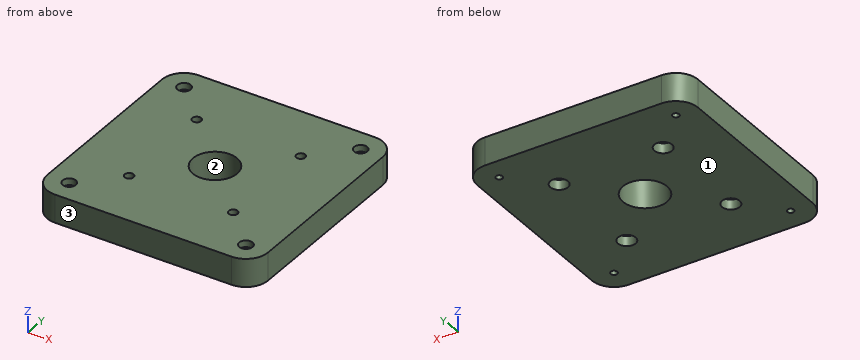
from build123d import *

# Parameters (mm, degrees)
SALIENTE_EXTRUIR4_START = 70
SALIENTE_EXTRUIR4_DEPTH = 12.7
CROQUIS8_R              = 3
CORTAR_EXTRUIR1_DEPTH   = 3
CROQUIS13_R             = 1.5
CORTAR_EXTRUIR4_DEPTH   = 30
CROQUIS16_R             = 10
CROQUIS16_R_2           = 2
CORTAR_EXTRUIR6_DEPTH   = 31
CROQUIS21_R             = 4
CORTAR_EXTRUIR12_DEPTH  = 4.5


with BuildPart() as part:
    # Croquis5 → Saliente-Extruir4 (new body)
    with BuildSketch(Plane.XY.offset(12.7).offset(SALIENTE_EXTRUIR4_START)):
        with BuildLine():
            Line((160, 0), (80, 0))
            ThreePointArc((80, 0), (72.928932188, 2.928932188), (70, 10))
            Line((70, 10), (70, 90))
            ThreePointArc((70, 90), (72.928932188, 97.071067812), (80, 100))
            Line((80, 100), (160, 100))
            ThreePointArc((160, 100), (167.071067812, 97.071067812), (170, 90))
            Line((170, 90), (170, 10))
            ThreePointArc((170, 10), (167.071067812, 2.928932188), (160, 0))
        make_face()
    extrude(amount=SALIENTE_EXTRUIR4_DEPTH)

    # Croquis8 → Cortar-Extruir1 (cut)
    with BuildSketch(Plane.XY.offset(95.4)):
        with Locations((80, 90)):
            Circle(CROQUIS8_R)
        with Locations((160, 90)):
            Circle(CROQUIS8_R)
        with Locations((160, 10)):
            Circle(CROQUIS8_R)
        with Locations((80, 10)):
            Circle(CROQUIS8_R)
    extrude(amount=-CORTAR_EXTRUIR1_DEPTH, mode=Mode.SUBTRACT)

    # Croquis13 → Cortar-Extruir4 (cut)
    with BuildSketch(Plane.XY.offset(95.4)):
        with Locations((80, 90)):
            Circle(CROQUIS13_R)
        with Locations((160, 90)):
            Circle(CROQUIS13_R)
        with Locations((160, 10)):
            Circle(CROQUIS13_R)
        with Locations((80, 10)):
            Circle(CROQUIS13_R)
    extrude(amount=-CORTAR_EXTRUIR4_DEPTH, mode=Mode.SUBTRACT)

    # Croquis16 → Cortar-Extruir6 (cut)
    with BuildSketch(Plane.XY.offset(95.4)):
        with Locations((120, 50)):
            Circle(CROQUIS16_R)
        with Locations((96.43, 73.57)):
            Circle(CROQUIS16_R_2)
        with Locations((143.57, 73.57)):
            Circle(CROQUIS16_R_2)
        with Locations((96.43, 26.43)):
            Circle(CROQUIS16_R_2)
        with Locations((143.57, 26.43)):
            Circle(CROQUIS16_R_2)
    extrude(amount=-CORTAR_EXTRUIR6_DEPTH, mode=Mode.SUBTRACT)

    # Croquis21 → Cortar-Extruir12 (cut)
    with BuildSketch(Plane(origin=(0, 0, 82.7), x_dir=(-1, 0, 0), z_dir=(0, 0, -1))):
        with Locations((-143.57, 73.57)):
            Circle(CROQUIS21_R)
        with Locations((-96.43, 73.57)):
            Circle(CROQUIS21_R)
        with Locations((-143.57, 26.43)):
            Circle(CROQUIS21_R)
        with Locations((-96.43, 26.43)):
            Circle(CROQUIS21_R)
    extrude(amount=-CORTAR_EXTRUIR12_DEPTH, mode=Mode.SUBTRACT)


solid = part.part
For this review, take the finished solid that the model builds, in its own axes (mm). Face numbers are marked on the shaded views. Round coordinates to 2 decimals unless told otherwise and drop trailing zeros. Write each loop counter-clockwise with the first axis right and the second up, starting at its lowest first coordinate (ties: lowest second). Pieces come first, ordered by that corner, then holes. Notation, with made-up numbers: (4.5, 7) - (62.5, 7) arc R30 ccw to (62.5, 43) - close; hole circle Ø3 at (41, -21). An arc over 180 degrees is marked (long way). Write item = value, one per line. Start each with the question number.
1. Consider section D-D on z = 85.25. Give the number of separate pieces and of enclosed holes in the cut face, plus the area to 3 significant figures.
2. Consider section B-B on y = 50. State the section outline as (x, z) points, plus the area to 3 significant figures.
3. Consider section A-A on x = 96.43. State the section outline as (y, z) points.
4. Consider section C-C on y = 73.57. State the section outline as (x, z) points.
5. For pin 1 Ø10.5 at (x, y) = (96.43, 73.57) entering from -Z; pin 2 Ø4 at (x, y) = (97, 73.5) entering from -Z; pin 3 Ø12 at (x, y) = (120, 50) entering from +Z; pin 4 Ø1.8 at (x, y) = (81, 10.5) entering from +Z, all flat-tipped, find the tip position at first contact; note any pin that passes through.
6. Wall thickness on L1, parallel to Y at x = 160, z = 93.9; L2, parallel to Y at x = 143.57, z = 86.3; L3, parallel to X at y = 25.5, z = 86.5: over which ranges is each line inside the solid? List them lowest first.
7. Draft analysis for pull direction Y (two halves, no side actions). For the marked faces 1, 2 and 3, state which applies: released by +Y, released by -Y, zero draft, split by the parting line, or undercut.
Evaluation:
q1.separate_pieces = 1
q1.enclosed_holes = 9
q1.area = 9,370 mm2
q2.outline = (70, 82.7) - (110, 82.7) - (110, 95.4) - (70, 95.4) - close; (130, 82.7) - (170, 82.7) - (170, 95.4) - (130, 95.4) - close
q2.area = 1,020 mm2
q3.outline = (0, 82.7) - (22.43, 82.7) - (22.43, 87.2) - (24.43, 87.2) - (24.43, 95.4) - (0, 95.4) - close; (28.43, 87.2) - (30.43, 87.2) - (30.43, 82.7) - (69.57, 82.7) - (69.57, 87.2) - (71.57, 87.2) - (71.57, 95.4) - (28.43, 95.4) - close; (75.57, 87.2) - (77.57, 87.2) - (77.57, 82.7) - (100, 82.7) - (100, 95.4) - (75.57, 95.4) - close
q4.outline = (70, 82.7) - (92.43, 82.7) - (92.43, 87.2) - (94.43, 87.2) - (94.43, 95.4) - (70, 95.4) - close; (98.43, 87.2) - (100.43, 87.2) - (100.43, 82.7) - (139.57, 82.7) - (139.57, 87.2) - (141.57, 87.2) - (141.57, 95.4) - (98.43, 95.4) - close; (145.57, 87.2) - (147.57, 87.2) - (147.57, 82.7) - (170, 82.7) - (170, 95.4) - (145.57, 95.4) - close
q5.pin_1 = 82.7
q5.pin_2 = 87.2
q5.pin_3 = through
q5.pin_4 = 92.4
q6.L1 = 0 to 7, 13 to 87, 93 to 100
q6.L2 = 0 to 22.43, 30.43 to 69.57, 77.57 to 100
q6.L3 = 70 to 92.54, 100.32 to 139.68, 147.46 to 170
q7.face_1 = zero draft
q7.face_2 = undercut
q7.face_3 = released by -Y
